```python
from build123d import *

# Parameters (mm, degrees)
F3_R          = 3
F4_DEPTH      = 25
F4_DEPTH_BACK = 25


with BuildPart() as f1:
    # F0 (on Front) → F1 (revolve)
    with BuildSketch(Plane.XZ):
        Polygon((-20, 0), (-6, 0), (0, 0), (6, 0), (18, 0), (25, 0), (25, 4), (-25, 3), (-25, 0), align=None)
    revolve(axis=Axis((1, 0, 0), (1, 0, 0)))

    # F0 (on Front) → F2 (revolve)
    with BuildSketch(Plane.XZ):
        with BuildLine():
            ThreePointArc((-30, 0), (-25, -5), (-20, 0))
            Line((-20, 0), (-25, 0))
            Line((-25, 0), (-30, 0))
        make_face()
        with BuildLine():
            Line((0, 0), (-6, 0))
            ThreePointArc((-6, 0), (0, -6), (6, 0))
            Line((6, 0), (0, 0))
        make_face()
        with BuildLine():
            Line((25, 0), (18, 0))
            ThreePointArc((18, 0), (25, -7), (32, 0))
            Line((32, 0), (25, 0))
        make_face()
    revolve(axis=Axis((1, 0, 0), (1, 0, 0)))

    # F3 (on Top) → F4 (cut, two sides)
    with BuildSketch(Plane.XY) as f4_sk:
        Circle(F3_R)
    extrude(amount=-F4_DEPTH, mode=Mode.SUBTRACT)
    extrude(f4_sk.sketch, amount=F4_DEPTH_BACK, mode=Mode.SUBTRACT)

    # F5 (on Front) → F6 (revolve)
    with BuildSketch(Plane.XZ):
        with BuildLine():
            Line((-27.5, 0), (-25, 0))
            Line((-25, 0), (-25, 35))
            add(Edge.make_bspline(
                [(-29.5, 6.5), (-28.6199930521, 6.710748409), (-25.1690403248, 7.5371996075), (-32.8021438158, 33.1401397633), (-26.9417712134, 34.537124263), (-25, 35)],
                knots=[0, 0, 0, 0, 0.1862478232, 0.7303719987, 1, 1, 1, 1], degree=3))
            Line((-29.5, 6.5), (-29.5, 4.5))
            Line((-29.5, 4.5), (-27.5, 4.5))
            Line((-27.5, 4.5), (-27.5, 0))
        make_face()
    revolve(axis=Axis((-25, 0, 17.5), (0, 0, 1)))


solid = f1.part
```
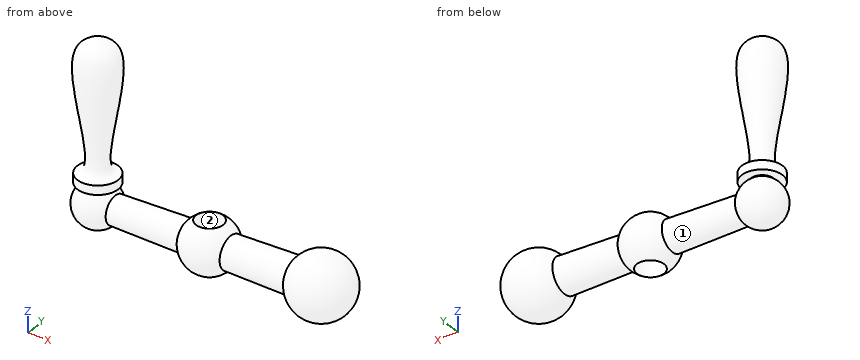
The listing builds one solid part. Answer for the finished solid, in the listing's coordinates (mm). Face numbers are marked on the shaded views. A direction names the side the tool comes from. Coordinates: 2 decimals unless noted, no trailing zeros. Loops run counter-clockwise (first coordinate to the right, second up) from the corner with the lowest first, then second, coordinate; pieces in that order, holes last. Notation, with made-up numbers: (-18.75, -15) - (29.25, -15) arc R15 ccw to (29.25, 12) - close; hole circle Ø11 at (-22.75, -14.75). An arc over 180 degrees is marked (long way). Use a Markdown table: item, result. Add a question column.
1) Find the intervals of material crossed by line 1 (X direction, y = 0, z = 2.5); line 2 (Y direction, x = 0, z = -1); line 3 (X direction, y = 0, z = -2.75), in increasing order.
2) For the marked faces 1 and 2, determine the directions among +Z, -Z, +X, -X, +Y, -Y from which every point of the face is accessible in a straight line to the end or side of a thin tool.
3) Given pin 1 (6 mm diameter, centred on x = -8.5, y = -5, fed in from +Z); pin 2 (6 mm diameter, centred on x = 13, y = 4.5, fed in from +Z); pin 3 (3.5 mm diameter, centred on x = 0, y = 0, fed in from +Z); pin 4 (2.5 mm diameter, centred on x = -26, y = 0.5, fed in from -Z), each flat-ended and moving along its own axis, determine where each tip first touches the part or whether it passes through.
4) The part is cut by section B-B, the plane x = 8. Give the vertices of the cut face in (y, z).
5) The part is cut by section A-A, the plane x = 0. Give the vertices of the cut face in (y, z).
6) The part is cut by section C-C, the plane x = -17.5. Give the vertices of the cut face in (y, z), and give its area (3 significant figures).
Here are the results:
| question | item | result |
|---|---|---|
| 1 | line 1 | x = -29.33 to -3, 3 to 31.54 |
| 1 | line 2 | y = -5.92 to -3, 3 to 5.92 |
| 1 | line 3 | x = -29.18 to -3, 3 to 31.44 |
| 2 | face 1 | none |
| 2 | face 2 | +Z, -Z |
| 3 | pin 1 | stops at z = 2.66 |
| 3 | pin 2 | stops at z = 3.45 |
| 3 | pin 3 | passes through |
| 3 | pin 4 | stops at z = -5 |
| 4 | outline | circle Ø7.32 at (0, 0) |
| 5 | outline | (-3, -5.2) - (-3, 5.2) arc R6 ccw to start; (3, -5.2) arc R6 ccw to (3, 5.2) - close |
| 6 | outline | circle Ø6.3 at (0, 0) |
| 6 | area | 31.2 mm^2 |
